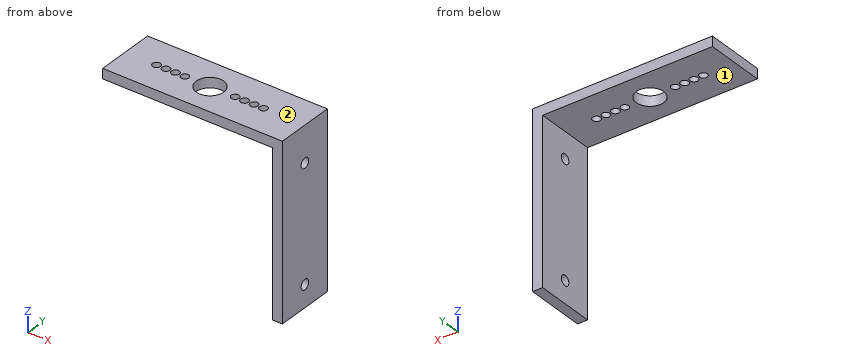
```python
from build123d import *

# Parameters (mm, degrees)
SKETCH1_W           = 53.975
SKETCH1_H           = 19.05
SKETCH1_R           = 1.25
SKETCH1_R_2         = 4.365625
BOSS_EXTRUDE1_DEPTH = 3.175
SKETCH2_W           = 55.245
SKETCH2_H           = 19.05
SKETCH2_R           = 1.5875
BOSS_EXTRUDE2_DEPTH = 3.175


with BuildPart() as part:
    # Sketch1 → Boss-Extrude1 (new body)
    with BuildSketch(Plane.XY):
        with Locations((26.9875, 9.525)):
            Rectangle(SKETCH1_W, SKETCH1_H)
        with Locations((34.9875114, 9.525)):
            Circle(SKETCH1_R, mode=Mode.SUBTRACT)
        with Locations((43.9874934, 9.525)):
            Circle(SKETCH1_R, mode=Mode.SUBTRACT)
        with Locations((37.9875054, 9.525)):
            Circle(SKETCH1_R, mode=Mode.SUBTRACT)
        with Locations((40.9874994, 9.525)):
            Circle(SKETCH1_R, mode=Mode.SUBTRACT)
        with Locations((18.9874886, 9.525)):
            Circle(SKETCH1_R, mode=Mode.SUBTRACT)
        with Locations((15.9874946, 9.525)):
            Circle(SKETCH1_R, mode=Mode.SUBTRACT)
        with Locations((12.9875006, 9.525)):
            Circle(SKETCH1_R, mode=Mode.SUBTRACT)
        with Locations((9.9875066, 9.525)):
            Circle(SKETCH1_R, mode=Mode.SUBTRACT)
        with Locations((26.9875, 9.525)):
            Circle(SKETCH1_R_2, mode=Mode.SUBTRACT)
    extrude(amount=BOSS_EXTRUDE1_DEPTH)

    # Sketch2 → Boss-Extrude2 (add)
    with BuildSketch(Plane(origin=(53.975, 0, 0), x_dir=(0, 0, -1), z_dir=(1, 0, 0))):
        with Locations((24.4475, 9.525)):
            Rectangle(SKETCH2_W, SKETCH2_H)
        with Locations((8.3185, 9.525)):
            Circle(SKETCH2_R, mode=Mode.SUBTRACT)
        with Locations((45.0215, 9.525)):
            Circle(SKETCH2_R, mode=Mode.SUBTRACT)
    extrude(amount=BOSS_EXTRUDE2_DEPTH)


solid = part.part
```
Input: part model. Units: mm. Frame: model coordinates. Face numbers are marked on the shaded views. A direction names the side the tool comes from. Give positions to 0.01 mm unless a question says otherwise; leave off trailing zeros. Order: outer loops, then holes, each group sorted by start corner. A loop starts at its lowest first (then second) coordinate and runs counter-clockwise, first axis right, second up.
1. Cut plane A-A (z = -45). Return loops of the section in (x, y) (3 decimals).
Computed:
outline: (53.975, 0) - (57.15, 0) - (57.15, 7.938) - (53.975, 7.938) - close; (53.975, 11.112) - (57.15, 11.112) - (57.15, 19.05) - (53.975, 19.05) - close
2. Cut plane B-B (y = 17.75). Return loops of the section in (x, z) (3 decimals).
Computed:
outline: (0, 0) - (53.975, 0) - (53.975, -52.07) - (57.15, -52.07) - (57.15, 3.175) - (0, 3.175) - close
3. Set-up query: the marked faces 1 and 2. Return all of +Z, -Z, +X, -X, +Y, -Y with unobstructed straight access to the full face (end or side cutting, diameter ignored); none if empty.
Computed:
face 1: -Z, -X, +Y, -Y
face 2: +Z, +X, -X, +Y, -Y
4. Pin query (flat end, axial travel): pin 1 Ø2 at (x, y) = (34.99, 9.52) entering from +Z; pin 2 Ø1.5 at (x, y) = (33, 15) entering from -Z; pin 3 Ø10 at (y, z) = (15, -20) entering from -X (3 decimals). Return the tip coordinate at first contact, or that it passes through.
Computed:
pin 1: passes through
pin 2: stops at z = 0
pin 3: stops at x = 53.975
5. Line query: probe 1 along X at (y, z) = (14.5, -49) (3 decimals); probe 2 along Z at (x, y) = (5.5, 10.5) (3 decimals). Output: solid intervals per line, ascending.
Computed:
probe 1: x = 53.975 to 57.15
probe 2: z = 0 to 3.175
6. Cut plane C-C (x = 16). Return loops of the section in (y, z) (3 decimals).
Computed:
outline: (0, 0) - (8.275, 0) - (8.275, 3.175) - (0, 3.175) - close; (10.775, 0) - (19.05, 0) - (19.05, 3.175) - (10.775, 3.175) - close
7. Cut plane D-D (x = 50.5). Return loops of the section in (y, z) (3 decimals).
Computed:
outline: (0, 0) - (19.05, 0) - (19.05, 3.175) - (0, 3.175) - close
